Build history of the part. All positions in model axes, mm. A direction names the side the tool comes from. Round coordinates to 2 decimals unless told otherwise and drop trailing zeros. Order: outer loops, then holes, each group sorted by start corner. A loop starts at its lowest first (then second) coordinate and runs counter-clockwise, first axis right, second up. Notation, with made-up numbers: (14, 51) -> (33, 51) arc R35 ccw to (33, 90) -> close; hole circle Ø6 at (15, 18). An arc over 180 degrees is marked (long way). Write item = value, one per line.
from build123d import *

# Parameters (mm, degrees)
F0_W     = 127
F0_H     = 76.2
F1_DEPTH = 76.2
F3_DEPTH = 127.001
F4_R     = 25.4
F6_DEPTH = 6.35


with BuildPart() as f1:
    # F0 (on Front) → F1 (new body)
    with BuildSketch(Plane.XZ):
        Rectangle(F0_W, F0_H)
    extrude(amount=F1_DEPTH)

    # F2 (on face) → F3 (cut, through all)
    with BuildSketch(Plane(origin=(-63.5, 0, 0), x_dir=(0, -1, 0), z_dir=(-1, 0, 0))):
        with BuildLine():
            ThreePointArc((14.3655382942, 38.1), (37.6635127669, 61.5633803993), (68.9486063382, 72.2670598849))
            Line((68.9486063382, 72.2670598849), (-52.0951251411, 60.1213361119))
            Line((-52.0951251411, 60.1213361119), (-33.0926589668, -48.5322624445))
            Line((-33.0926589668, -48.5322624445), (48.5539544729, -67.162540312))
            ThreePointArc((48.5539544729, -67.162540312), (29.1590805148, -55.3377136177), (14.3655382942, -38.1))
            Line((14.3655382942, -38.1), (0, -38.1))
            Line((0, -38.1), (0, 38.1))
            Line((0, 38.1), (14.3655382942, 38.1))
        make_face()
        with BuildLine():
            ThreePointArc((14.3655382942, -38.1), (3.5700429957, 0), (14.3655382942, 38.1))
            Line((14.3655382942, 38.1), (0, 38.1))
            Line((0, 38.1), (0, -38.1))
            Line((0, -38.1), (14.3655382942, -38.1))
        make_face()
    extrude(amount=-F3_DEPTH, mode=Mode.SUBTRACT)

    # F4
    f4_edges = [f1.edges().sort_by_distance(p)[0] for p in [
        (-63.5, -45.282769, 38.1),
        (63.5, -45.282769, 38.1),
        (-63.5, -45.282769, -38.1),
        (63.5, -45.282769, -38.1),
        (63.5, -3.570043, 0),
        (-63.5, -3.570043, 0),
        (0, -14.365538, -38.1),
        (0, -14.365538, 38.1),
    ]]
    fillet(f4_edges, radius=F4_R)

    # F5 (on face) → F6 (cut)
    with BuildSketch(Plane.XZ.offset(76.2)):
        with BuildLine():
            Line((57.1500010133, -12.7), (57.1500010133, 12.7))
            ThreePointArc((57.1500010133, 12.7), (51.5703848981, 26.1703848981), (38.1, 31.7500010133))
            Line((38.1, 31.7500010133), (-38.1, 31.7500010133))
            ThreePointArc((-38.1, 31.7500010133), (-51.5703848981, 26.1703848981), (-57.1500010133, 12.7))
            Line((-57.1500010133, 12.7), (-57.1500010133, -12.7))
            ThreePointArc((-57.1500010133, -12.7), (-51.5703848981, -26.1703848981), (-38.1, -31.7500010133))
            Line((-38.1, -31.7500010133), (38.1, -31.7500010133))
            ThreePointArc((38.1, -31.7500010133), (51.5703848981, -26.1703848981), (57.1500010133, -12.7))
        make_face()
    extrude(amount=-F6_DEPTH, mode=Mode.SUBTRACT)


solid = f1.part
Q1. Mould opens along X. For faces 3 (the face through (55.86, -53.77, -30.86)), 4 (the face through (-0.53, -15.17, -32.79)), 5 (the face through (57.15, -73, 0)) say: released by +X, released by -X, zero draft, split by the parting line, or undercut.
Check values:
face_3 = released by +X
face_4 = zero draft
face_5 = undercut
Q2. Probe probe 1 along X at (y, z) = (-71, 3); probe 2 along Z at (x, y) = (-2.5, -72); probe 3 along X at (y, z) = (-26.5, 24.5). List the from-to ranges inside material, lowest first.
Check values:
probe_1 = -63.5 to -57.15, 57.15 to 63.5
probe_2 = -38.1 to -31.75, 31.75 to 38.1
probe_3 = -60.2 to 60.2
Q3. Cut at C-C, the plane z = 33.5. List the corners of the cut face in (x, y), and give its area (3 significant figures).
Check values:
outline = (-52.68, -76.2) -> (52.68, -76.2) -> (52.68, -30.71) arc R14.58 ccw to (38.1, -16.13) -> (-38.1, -16.13) arc R14.58 ccw to (-52.68, -30.71) -> close
area = 6,240 mm²
Q4. Cut at B-B, the plane y = -46. List the corners of the cut face in (x, z), and give its area (3 significant figures).
Check values:
outline = (-63.5, -12.7) arc R25.4 ccw to (-38.1, -38.1) -> (38.1, -38.1) arc R25.4 ccw to (63.5, -12.7) -> (63.5, 12.7) arc R25.4 ccw to (38.1, 38.1) -> (-38.1, 38.1) arc R25.4 ccw to (-63.5, 12.7) -> close
area = 9,120 mm²
Q5. Which spindle directions (+Z, -Z, +X, -X, +Y, -Y) get a long thin tool onto all of the face, cutting with end or side? Do faces 1 (the face through (-57.15, -73, 0)), 2 (the face through (63.5, -52, 0)). Say none if no direction does.
Check values:
face_1 = -Y
face_2 = +Z, -Z, +X, +Y, -Y
Q6. Flat gauge pins, fed straight in: pin 1 (3 mm diameter, centred on x = -14, z = -16, fed in from +Y); pin 2 (1 mm diameter, centred on x = 5.5, y = -11, fed in from +Z); pin 3 (8 mm diameter, centred on x = 22, z = -20, fed in from +Y). Where does each tip first touch, or does it go through?
Check values:
pin_1 = -5.03
pin_2 = 29.32
pin_3 = -5.35
Q7. Cut at D-D, the plane x = 44. List the corners of the cut face in (y, z), and give its area (3 significant figures).
Check values:
outline = (-76.2, -37.41) -> (-30.71, -37.41) arc R24.71 ccw to (-6.91, -19.34) arc R71.94 ccw to (-6.91, 19.34) arc R24.71 ccw to (-30.71, 37.41) -> (-76.2, 37.41) -> (-76.2, 30.81) -> (-69.85, 30.81) -> (-69.85, -30.81) -> (-76.2, -30.81) -> close
area = 4,640 mm²
Q8. Cut at A-A, the plane x = -25. List the corners of the cut face in (y, z).
Check values:
outline = (-76.2, -38.1) -> (-30.71, -38.1) arc R25.4 ccw to (-6.25, -19.53) arc R72.63 ccw to (-6.25, 19.53) arc R25.4 ccw to (-30.71, 38.1) -> (-76.2, 38.1) -> (-76.2, 31.75) -> (-69.85, 31.75) -> (-69.85, -31.75) -> (-76.2, -31.75) -> close
